from build123d import *


with BuildPart() as part:
    # Sketch1 → Revolve1 (revolve)
    with BuildSketch(Plane.XY, mode=Mode.PRIVATE) as revolve1_sk:
        with BuildLine():
            Line((0, 0), (47.5, 0))
            Line((47.5, 0), (47.5, 8))
            Line((47.5, 8), (43.5, 8))
            Line((43.5, 8), (43.5, 15))
            Line((43.5, 15), (47.5, 15))
            Line((47.5, 15), (47.5, 305.5))
            ThreePointArc((47.5, 305.5), (45, 308), (47.5, 310.5))
            Line((47.5, 310.5), (47.5, 332))
            Line((47.5, 332), (25, 332))
            Line((25, 332), (25, 82))
            Line((25, 82), (0, 82))
            Line((0, 82), (0, 0))
        make_face()
    revolve(revolve1_sk.sketch.rotate(Axis((0, 0, 0), (0, 1, 0)), 90), axis=Axis((0, 0, 0), (0, 1, 0)))


solid = part.part
Model file for the job. Use its own axes, mm. A direction names the side the tool comes from. Give positions to 0.01 mm unless a question says otherwise; leave off trailing zeros. Order: outer loops, then holes, each group sorted by start corner. A loop starts at its lowest first (then second) coordinate and runs counter-clockwise, first axis right, second up. Notation, with made-up numbers: M 75,-7.75 L 83,-7.75 A30 ccw 83,18.25 Z; hole C -8.5,80.5 d4. An arc over 180 degrees is marked long. Put each result on its own line as item: value. Start each with the question number.
(1) Tool access for faces 1 (the face through (-7.509, 205.25, -23.846)), 2 (the face through (38.5, 8, -20.9)), 3 (the face through (46.37, 162.28, 10.3)): list every direction of +Z, -Z, +X, -X, +Y, -Y with a clear straight run to the whole face (end or side of a thin tool).
(2) Pin check, flat tips, straight feed: pin 1 Ø4 at (x, z) = (9, -21) entering from +Y; pin 2 Ø10 at (x, y) = (29.5, 143.5) entering from +Z; pin 3 Ø1.5 at (x, y) = (-16.5, 119.5) entering from -Z. Stop position of each tip, or through.
(3) Band-saw the part on B-B on y = 192. Give the cut face in (x, z), then the cut area to 3 significant figures.
(4) Band-saw the part on D-D on y = 49.5. Give the cut face in (x, z), then the cut area to 3 significant figures.
(5) Drill centre lines: L1, parallel to Y at x = -17.5, z = -40.5; L2, parallel to X at y = 253, z = 0; L3, parallel to Y at x = -19.5, z = -4.5. Where is each one in solid material? Low to high. Write a range as [from, to].
(6) Pull direction Z, two halves, no side cores. Call faces 4 (the face through (-1, 0, -1)), 5 (the face through (0, 82, 0)), 6 (the face through (46.37, 4.06, 10.3)): released by +Z, released by -Z, zero draft, split by the parting line, or undercut.
(7) Band-saw the part on C-C on z = 0. Give the cut face in (x, y), then the cut area to 3 significant figures.
(8) Band-saw the part on A-A on x = 0. Give the cut face in (y, z), then the cut area to 3 significant figures.
Results below:
1. face 1: +Y
1. face 2: none
1. face 3: +Y, -Y
2. pin 1: stops at y = 82
2. pin 2: stops at z = 40.69
2. pin 3: stops at z = -44.81
3. outline: C 0,0 d95; hole C 0,0 d50
3. area: 5,120 mm2
4. outline: C 0,0 d95
4. area: 7,090 mm2
5. L1: y = [0, 8], [15, 332]
5. L2: x = [-47.5, -25], [25, 47.5]
5. L3: y = [0, 82]
6. face 4: zero draft
6. face 5: undercut
6. face 6: split by the parting line
7. outline: M -47.5,0 L 47.5,0 L 47.5,8 L 43.5,8 L 43.5,15 L 47.5,15 L 47.5,305.5 A2.5 cw 47.5,310.5 L 47.5,332 L 25,332 L 25,82 L -25,82 L -25,332 L -47.5,332 L -47.5,310.5 A2.5 cw -47.5,305.5 L -47.5,15 L -43.5,15 L -43.5,8 L -47.5,8 Z
7. area: 19,000 mm2
8. outline: M 0,-47.5 L 8,-47.5 L 8,-43.5 L 15,-43.5 L 15,-47.5 L 305.5,-47.5 A2.5 cw 310.5,-47.5 L 332,-47.5 L 332,-25 L 82,-25 L 82,25 L 332,25 L 332,47.5 L 310.5,47.5 A2.5 cw 305.5,47.5 L 15,47.5 L 15,43.5 L 8,43.5 L 8,47.5 L 0,47.5 Z
8. area: 19,000 mm2
